Could you check a few things on this drawing? It's one solid part, dimensions in mm from its lowest x, y, z. A direction names the side the tool comes from. Round coordinates to 2 decimals unless told otherwise and drop trailing zeros. Order: outer loops, then holes, each group sorted by start corner. A loop starts at its lowest first (then second) coordinate and runs counter-clockwise, first axis right, second up.
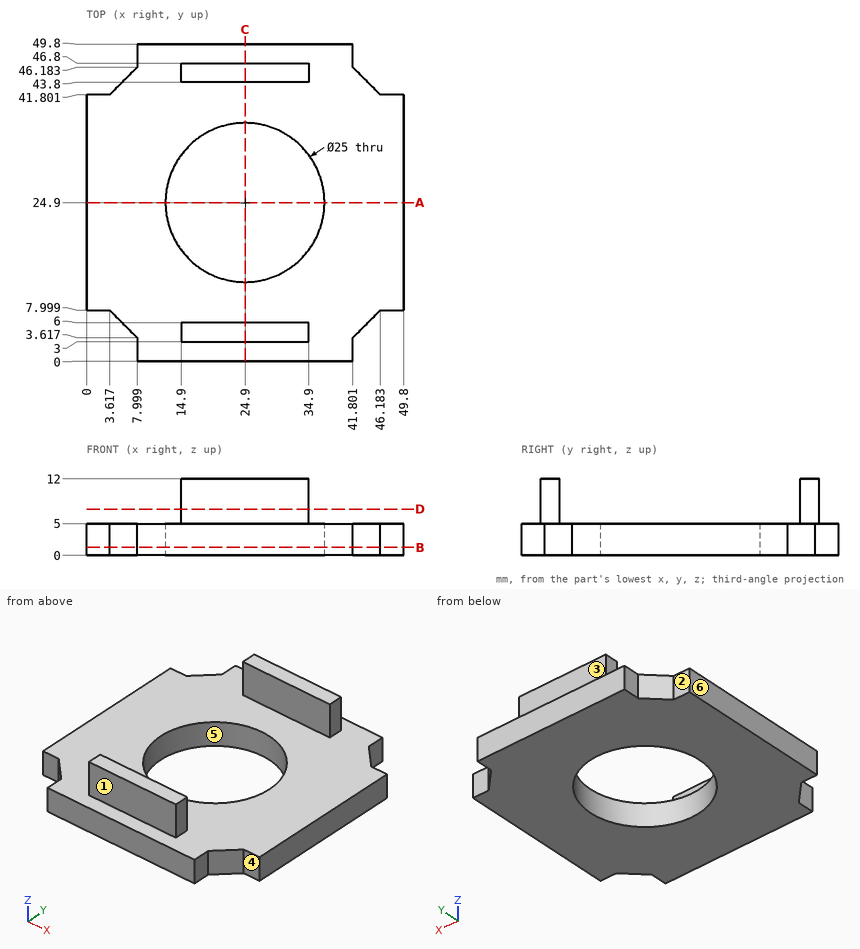
(1) On a 3-axis mill with a long thin cutter (end or side, diameter ignored), from which of +Z, -Z, +X, -X, +Y, -Y can I reach the whole of each face in a straight line? I mean the marked faces 1, 2 and 3. Say none if no direction works.
(2) Please list where these lines run through material, in increasing order: probe 1 along Y at (x, z) = (22, 11); probe 2 along Y at (x, z) = (24.9, 3.15); probe 3 along Z at (x, y) = (45, 19).
(3) I want a section at C-C, the plane x = 24.9. List the corners of the cut face in (y, z) for me, plus the area to 3 significant figures.
(4) I want a section at A-A, the plane y = 24.9. List the corners of the cut face in (x, z) for me, plus the area to 3 significant figures.
(5) If we mould it in two halves opening along Y, with no side actions, what happens to the marked faces 4, 5 and 6? For each: pulls with the +Y half, pulls with the -Y half, needs draft (parallel to the pull), parting line crosses it, or undercut.
(6) I want a section at B-B, the plane z = 1.25. List the corners of the cut face in (x, y) for me.
(7) I'm going to push flat-ended pins straight in: pin 1 Ø1.8 at (y, z) = (48.5, 3) entering from +X; pin 2 Ø1.5 at (y, z) = (44.5, 9) entering from -X; pin 3 Ø1.1 at (x, z) = (48.5, 2.5) entering from -Y; pin 4 Ø1.5 at (x, y) = (35, 28.5) entering from +Z. Where does each tip first touch, or does it pass through?
(8) I want a section at D-D, the plane z = 7.25. List the corners of the cut face in (x, y) for me, plus the area to 3 significant figures.
Ans:
1. face 1: +Z, +X, -X, -Y
1. face 2: +Z, -Z, -X, +Y
1. face 3: +Z, +X, -X, +Y
2. probe 1: y = 3 to 6, 43.8 to 46.8
2. probe 2: y = 0 to 12.4, 37.4 to 49.8
2. probe 3: z = 0 to 5
3. outline: (0, 0) - (12.4, 0) - (12.4, 5) - (6, 5) - (6, 12) - (3, 12) - (3, 5) - (0, 5) - close; (37.4, 0) - (49.8, 0) - (49.8, 5) - (46.8, 5) - (46.8, 12) - (43.8, 12) - (43.8, 5) - (37.4, 5) - close
3. area: 166 mm2
4. outline: (0, 0) - (12.4, 0) - (12.4, 5) - (0, 5) - close; (37.4, 0) - (49.8, 0) - (49.8, 5) - (37.4, 5) - close
4. area: 124 mm2
5. face 4: pulls with the -Y half
5. face 5: undercut
5. face 6: needs draft
6. outline: (0, 8) - (3.62, 8) - (8, 3.62) - (8, 0) - (41.8, 0) - (41.8, 3.62) - (46.18, 8) - (49.8, 8) - (49.8, 41.8) - (46.18, 41.8) - (41.8, 46.18) - (41.8, 49.8) - (8, 49.8) - (8, 46.18) - (3.62, 41.8) - (0, 41.8) - close; hole circle Ø25 at (24.9, 24.9)
7. pin 1: stops at x = 41.8
7. pin 2: stops at x = 14.9
7. pin 3: stops at y = 8
7. pin 4: passes through
8. outline: (14.9, 3) - (34.9, 3) - (34.9, 6) - (14.9, 6) - close; (14.9, 43.8) - (34.9, 43.8) - (34.9, 46.8) - (14.9, 46.8) - close
8. area: 120 mm2
